Read the model definition and answer for the solid it produces. Units are mm, in the model's axes. A direction names the side the tool comes from. Coordinates: 2 decimals unless noted, no trailing zeros. Write each loop counter-clockwise with the first axis right and the second up, starting at its lowest first coordinate (ties: lowest second). Pieces come first, ordered by that corner, then holes. Notation, with made-up numbers: (43.25, 46) -> (65.25, 46) arc R18 cw to (65.25, 51) -> close; hole circle Ø11 at (-10, -35.5). An arc over 180 degrees is marked (long way). Answer as a JSON object with one key per item and string values. Group by question number.
(1) Find section D-D (z = -44.5). Give the vertices of the cut face in (x, y), then the cut area to 3 significant figures.
(2) Straight lines are drawn through the part: L1, parallel to X at y = 5.5, z = -4; L2, parallel to Z at x = 79, y = 7.5; L3, parallel to X at y = 6.75, z = -48. For each, find the intervals that lie inside material, in ascending order.
(3) For a pull along Z with two mould halves and no side action, classify faces 1 (the face through (8, 5, -38.386)), 2 (the face through (40, 9.5, -51)), 3 (the face through (50, 1.5, -15)) as +Z half, -Z half, draft (parallel to the pull), parting line (faces both ways), or undercut.
(4) Find section A-A (y = 5.5). Count the separate pieces of the cut face and the enclosed holes in it, then the cut area to 3 significant figures.
(5) Flat-ended cylindrical pins translate along their axes: P1, Ø10, axis at x = 18.5, z = -21, coming from the +Y side; P2, Ø1.5, axis at x = 26.5, y = 7.5, coming from the -Z side; P3, Ø2.5, axis at x = 85, y = 5, coming from the +Z side. Find the tip coordinate at first contact, or state that the pin passes through.
(6) Find section C-C (x = 80). Give the vertices of the cut face in (y, z), then the cut area to 3 significant figures.
(7) Find section B-B (z = -15). Give the vertices of the cut face in (x, y), then the cut area to 3 significant figures.
(8) Which of the six approach directions +Z, -Z, +X, -X, +Y, -Y give full straight-line access (tool end or side, diameter ignored) to faces 4 (the face through (39, 5, -4.059)), 5 (the face through (95.312, 5, -3)), 6 (the face through (77.814, 5, -51)), 7 (the face through (66, 5, -53.163))?
from build123d import *

# Parameters (mm, degrees)
SKETCH1_W           = 102
SKETCH1_H           = 53.5
BOSS_EXTRUDE1_DEPTH = 1.5
SKETCH2_W           = 14.952348819
SKETCH2_H           = 9.85729203
BOSS_EXTRUDE2_DEPTH = 8
SKETCH3_W           = 26.751318109
SKETCH3_H           = 4.056156536
SKETCH3_W_2         = 22.308860949
SKETCH3_W_3         = 17.497554299
SKETCH3_W_4         = 3.694182794
SKETCH3_H_2         = 49.772168178
SKETCH3_W_5         = 21.695691939
SKETCH3_H_3         = 2.671784729
SKETCH3_W_6         = 19.752122819
SKETCH3_W_7         = 20.420069002
BOSS_EXTRUDE3_DEPTH = 8
SKETCH4_W           = 17.576678325
SKETCH4_H           = 17.576678325
BOSS_EXTRUDE4_DEPTH = 1


with BuildPart() as part:
    # Sketch1 → Boss-Extrude1 (new body)
    with BuildSketch(Plane(origin=(0, 0, 0), x_dir=(1, 0, 0), z_dir=(0, 1, 0))):
        with Locations((51, 26.75)):
            Rectangle(SKETCH1_W, SKETCH1_H)
    extrude(amount=BOSS_EXTRUDE1_DEPTH)

    # Sketch2 → Boss-Extrude2 (add)
    with BuildSketch(Plane(origin=(0, 1.5, 0), x_dir=(-1, 0, 0), z_dir=(0, 1, 0))):
        with Locations((-7.47617441, -43.314315473)):
            Rectangle(SKETCH2_W, SKETCH2_H)
    extrude(amount=BOSS_EXTRUDE2_DEPTH)

    # Sketch3 → Boss-Extrude3 (add)
    with BuildSketch(Plane(origin=(0, 1.5, 0), x_dir=(-1, 0, 0), z_dir=(0, 1, 0))):
        with Locations((-39.507531481, -51.135226796)):
            Rectangle(SKETCH3_W, SKETCH3_H)
        with Locations((-65.389673188, -51.135226796)):
            Rectangle(SKETCH3_W_2, SKETCH3_H)
        with Locations((-86.563053436, -51.135226796)):
            Rectangle(SKETCH3_W_3, SKETCH3_H)
        with Locations((-99.154840724, -28.277220975)):
            Rectangle(SKETCH3_W_4, SKETCH3_H_2)
        with Locations((-84.463984616, -2.723190704)):
            Rectangle(SKETCH3_W_5, SKETCH3_H_3)
        with Locations((-62.02250134, -2.723190704)):
            Rectangle(SKETCH3_W_6, SKETCH3_H_3)
        with Locations((-39.2646207, -2.723190704)):
            Rectangle(SKETCH3_W_7, SKETCH3_H_3)
    extrude(amount=BOSS_EXTRUDE3_DEPTH)

    # Sketch4 → Boss-Extrude4 (add)
    with BuildSketch(Plane(origin=(0, 1.5, 0), x_dir=(-1, 0, 0), z_dir=(0, 1, 0))):
        with Locations((-56.842771916, -27.377738511)):
            Rectangle(SKETCH4_W, SKETCH4_H)
    extrude(amount=BOSS_EXTRUDE4_DEPTH)


solid = part.part
Results below:
{
 "1": {"outline": "(0, 0) -> (102, 0) -> (102, 1.5) -> (101, 1.5) -> (101, 9.5) -> (97.31, 9.5) -> (97.31, 1.5) -> (14.95, 1.5) -> (14.95, 9.5) -> (0, 9.5) -> close", "area": "302 mm2"},
 "2": {"L1": "x = 29.05 to 49.47, 52.15 to 71.9, 73.62 to 95.31, 97.31 to 101", "L2": "z = -53.16 to -49.11, -4.06 to -1.39", "L3": "x = 0 to 14.95, 97.31 to 101"},
 "3": {"face 1": "+Z half", "face 2": "draft", "face 3": "undercut"},
 "4": {"separate pieces": "8", "enclosed holes": "0", "area": "767 mm2"},
 "5": {"P1": "stops at y = 1.5", "P2": "stops at z = -53.16", "P3": "stops at z = -1.39"},
 "6": {"outline": "(0, -53.5) -> (1.5, -53.5) -> (1.5, -53.16) -> (9.5, -53.16) -> (9.5, -49.11) -> (1.5, -49.11) -> (1.5, -4.06) -> (9.5, -4.06) -> (9.5, -1.39) -> (1.5, -1.39) -> (1.5, 0) -> (0, 0) -> close", "area": "134 mm2"},
 "7": {"outline": "(0, 0) -> (102, 0) -> (102, 1.5) -> (101, 1.5) -> (101, 9.5) -> (97.31, 9.5) -> (97.31, 1.5) -> (0, 1.5) -> close", "area": "183 mm2"},
 "8": {"face 4": "-X, +Y", "face 5": "+Z, -Z, +Y", "face 6": "-Z, +Y", "face 7": "-Z, +X, -X, +Y"}
}
